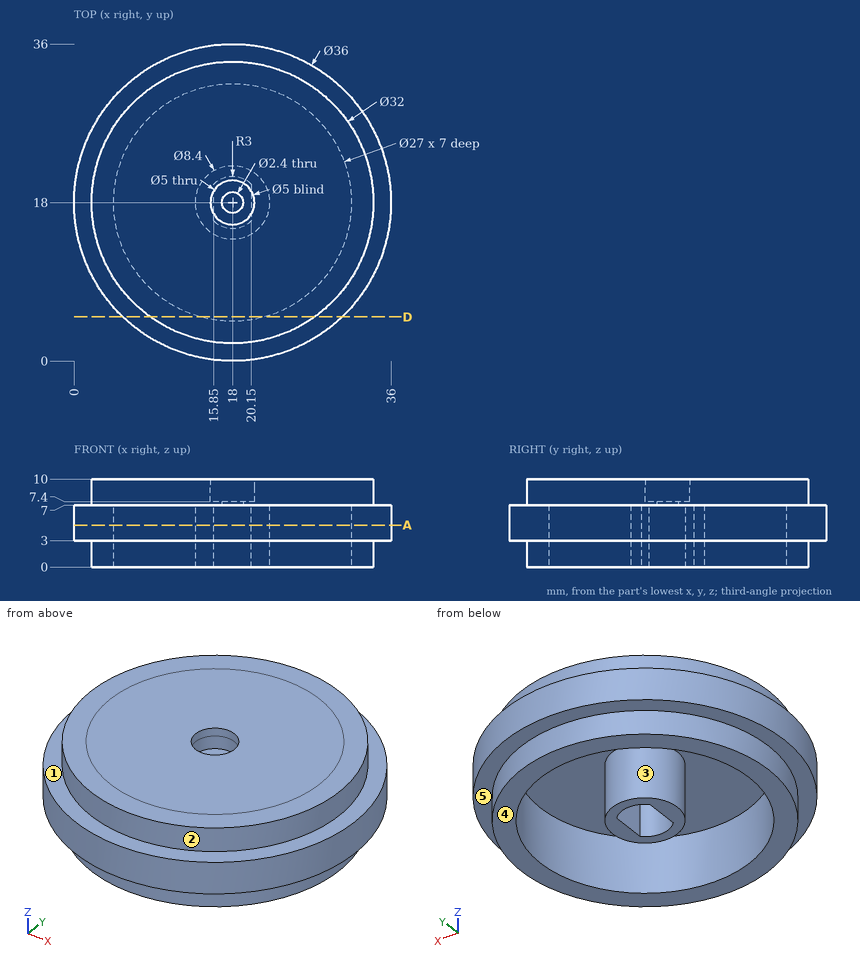
Input: dimensioned drawing with shaded views. Units: mm. Origin: part minimum x, y, z. A direction names the side the tool comes from. Coordinates: 2 decimals unless noted, no trailing zeros. Loops run counter-clockwise (first coordinate to the right, second up) from the corner with the lowest first, then second, coordinate; pieces in that order, holes last. Notation, with made-up numbers: M 75,-2.75 L 112,-2.75 A29 ccw 112,35.25 Z; hole C -4.75,32 d6. An arc over 180 degrees is marked long. One line per item, written item: value.
(1) Pull-direction query (Y, two-part tool) for the marked faces 1, 2 and 3; classes: +Y half, -Y half, draft (parallel to the pull), parting line (faces both ways), or undercut.
Filled in:
face 1: draft
face 2: parting line
face 3: undercut
(2) Section D-D (y = 5). Output: boundary loops of the cut face in (x, z).
Filled in:
outline: M 5.55,3 L 8.67,3 L 8.67,0 L 14.36,0 L 14.36,7 L 21.64,7 L 21.64,0 L 27.33,0 L 27.33,3 L 30.45,3 L 30.45,7 L 27.33,7 L 27.33,10 L 8.67,10 L 8.67,7 L 5.55,7 Z
(3) Pin query (flat end, axial travel): pin 1 (6 mm diameter, centred on x = 18, y = 18, fed in from +Z); pin 2 (2 mm diameter, centred on x = 12.5, z = 5.5, fed in from +Y); pin 3 (2 mm diameter, centred on x = 8, y = 24, fed in from -Z); pin 4 (1.3 mm diameter, centred on y = 17, z = 2, fed in from +X). Return the tip coordinate at first contact, or that it passes through.
Filled in:
pin 1: z = 10
pin 2: y = 35.43
pin 3: z = 7
pin 4: x = 34
(4) Line query: line 1 along Y through (x, z) = (18, 7.3); line 2 along Y through (x, z) = (18, 9); line 3 along Y through (x, z) = (20.5, 4.25). Output: solid intervals per line, ascending. Write a range as from..to.
Filled in:
line 1: 2..16.8, 19.2..34
line 2: 2..15.5, 20.5..34
line 3: 0.17..4.73, 14.63..21.37, 31.27..35.83
(5) Reachability of the marked faces 4 and 5 from +Z, -Z, +X, -X, +Y, -Y: full face, straight path, thin tool, end or side. Return the list, or none.
Filled in:
face 4: -Z, +X, -X, +Y, -Y
face 5: -Z
(6) Section A-A (z = 4.75). Output: boundary loops of the cut face in (x, y).
Filled in:
outline: C 18,18 d36; C 18,18 d8.4; hole C 18,18 d27; hole M 15.85,15.91 A3 ccw 20.15,15.91 L 20.15,20.09 A3 ccw 15.85,20.09 Z
